Autodesk Inventor part; units mm, degrees
ref_plane "YZ Plane" through (0, 0, 0) normal (1, 0, 0) x (0, 1, 0)
ref_plane "XZ Plane" through (0, 0, 0) normal (0, 1, 0) x (-1, 0, 0)
ref_plane "XY Plane" through (0, 0, 0) normal (0, 0, 1) x (1, 0, 0)
sketch "Sketch1" plane through (0, 0, 0) normal (0, 1, 0) x (-1, 0, 0)
  circle A0 centre (0, 0) radius 32
  line L0 (27.5, 0) -> (-27.5, 0) construction
  circle A1 centre (27.5, 0) radius 3.5
  circle A2 centre (-27.5, 0) radius 3.5
  line L1 (26, 32) -> (-26, 32)
  line L2 (-26, 32) -> (-26, -32)
  line L3 (-26, -32) -> (26, -32)
  line L4 (26, -32) -> (26, 32)
  line L5 (26, 32) -> (-26, -32) construction
  line L6 (-26, 32) -> (26, -32) construction
  line L7 (0, -32) -> (0, -13) construction
  line L8 (7.5, -32) -> (7.5, -13)
  line L9 (-7.5, -13) -> (-7.5, -32)
  arc A3 (-7.5, -32) -> (7.5, -32) centre (0, -32) ccw
  arc A4 (7.5, -13) -> (-7.5, -13) centre (0, -13) ccw
  line L10 (-28.2666, 32) -> (28.2666, 32)
  line L11 (28.2666, 32) -> (28.2666, 15)
  line L12 (28.2666, 15) -> (-28.2666, 15)
  line L13 (-28.2666, 15) -> (-28.2666, 32)
  point P0 (0, -22.5)
  point P1 (0, -5.5)
  point P2 (31, 0)
  point P3 (-31, 0)
  point P4 (-7.5, -31.1087)
  point P5 (7.5, -31.1087)
  dimension "d0" = 64
  dimension "d1" = 55
  dimension "d2" = 7
  dimension "d3" = 7
  dimension "d4" = 52
  dimension "d5" = 15
  dimension "d6" = 5.5
  dimension "d13" = 15
extrude "Extrusion1" add sketch "Sketch1" along normal blind 1 contours A0 L4 A1 L12 | A0 L8 A4 L9 L2 A2 L12 L4 A1 | L2 A2 A0 L12
fillet "Fillet1" radius 1 4 edges at (-7.5, 0.5, -31.1087) (7.5, 0.5, -31.1087) (-28.2666, 0.5, 15) (28.2666, 0.5, 15)
chamfer "Chamfer1" distance 0.25 angle 45 20 edges at (-24, 0, 0) (-24, 1, 0) (29.3193, 1, -12.8211) (7.8976, 1, -30.6101) (7.5, 1, -21.406) (0, 1, -5.5) (-7.5, 1, -21.406) (-7.8976, 1, -30.6101) (-29.3193, 1, -12.8211) (-29.3193, 0, -12.8211) (-7.8976, 0, -30.6101) (-7.5, 0, -21.406) (0, 0, -5.5) (7.5, 0, -21.406) (7.8976, 0, -30.6101) (29.3193, 0, -12.8211) (31, 0, 0) (31, 1, 0) (0, 0, 15) (0, 1, 15)
properties part number "Battery Cover"
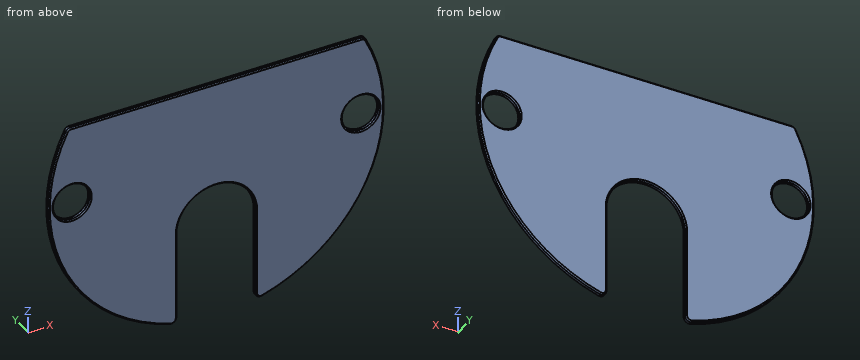
Can you work these out from the model? Positions are in its coordinate system, mm. Give positions to 0.01 mm unless a question says otherwise; leave off trailing zeros. Write each loop counter-clockwise with the first axis right and the second up, starting at its lowest first coordinate (ties: lowest second). Pieces come first, ordered by that corner, then holes. Notation, with made-up numbers: (22, 54) -> (67, 54) arc R12 ccw to (67, 63) -> close; hole circle Ø9 at (68, 65). An arc over 180 degrees is marked (long way). Write item = value, one per line.
(1) I need wall thicknesses on probe 1 along X at (y, z) = (0.55, 0); probe 2 along Z at (x, y) = (-25, 0.6); probe 3 along X at (y, z) = (0.6, -17). Which ranges of each line are inside material? Lowest first, please. Write a range as from..to.
Worked out:
probe_1 = -32..-31, -24..24, 31..32
probe_2 = -19.97..-2.45, 2.45..15
probe_3 = -27.11..-7.5, 7.5..27.11
(2) Suppose I cut it at A-A on y = 0.55. Write out the boundary of the cut face in (x, z).
Worked out:
outline = (-28.55, 14.45) arc R32 ccw to (-8.77, -30.77) arc R1 ccw to (-7.5, -29.81) -> (-7.5, -13) arc R7.5 cw to (7.5, -13) -> (7.5, -29.81) arc R1 ccw to (8.77, -30.77) arc R32 ccw to (28.55, 14.45) arc R1 ccw to (27.66, 15) -> (-27.66, 15) arc R1 ccw to start; hole circle Ø7 at (-27.5, 0); hole circle Ø7 at (27.5, 0)
(3) I'm going to push a flat-ended pin straight in: P1, Ø6.5, axis at x = 27.5, z = 0, coming from the +Y side. Where does the tip first touch, or does it pass through?
Worked out:
P1 = through
(4) Suppose I cut it at B-B on z = 0. Write out the boundary of the cut face in (x, y).
Worked out:
outline = (-32, 0.25) -> (-31.75, 0) -> (-31.25, 0) -> (-31, 0.25) -> (-31, 0.75) -> (-31.25, 1) -> (-31.75, 1) -> (-32, 0.75) -> close; (-24, 0.25) -> (-23.75, 0) -> (23.75, 0) -> (24, 0.25) -> (24, 0.75) -> (23.75, 1) -> (-23.75, 1) -> (-24, 0.75) -> close; (31, 0.25) -> (31.25, 0) -> (31.75, 0) -> (32, 0.25) -> (32, 0.75) -> (31.75, 1) -> (31.25, 1) -> (31, 0.75) -> close
(5) Suppose I cut it at C-C on x = 0. Write out the boundary of the cut face in (y, z).
Worked out:
outline = (0, -5.25) -> (0.25, -5.5) -> (0.75, -5.5) -> (1, -5.25) -> (1, 14.75) -> (0.75, 15) -> (0.25, 15) -> (0, 14.75) -> close
